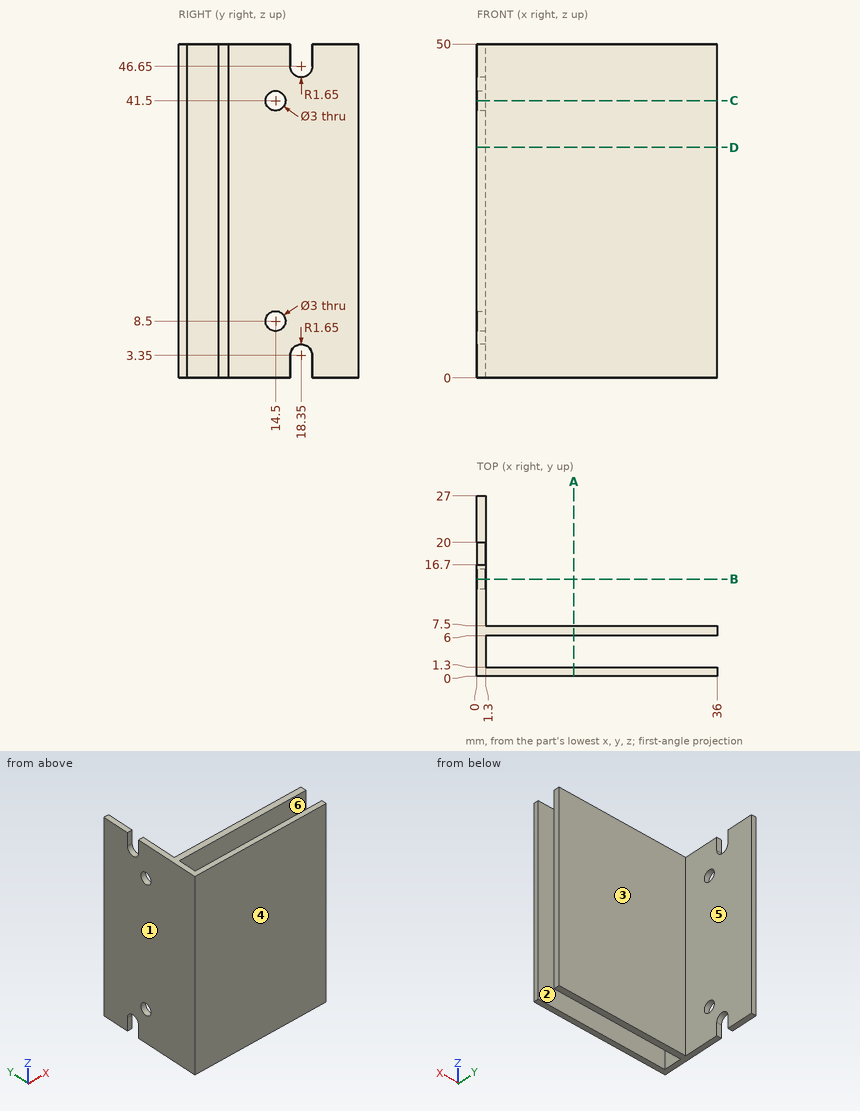
Answer from the drawing. Dimensions are ordinates in mm from the lowest x, y and z of the part. A direction names the side the tool comes from. Round coordinates to 2 decimals unless told otherwise and drop trailing zeros. Loops run counter-clockwise (first coordinate to the right, second up) from the corner with the lowest first, then second, coordinate; pieces in that order, holes last. Notation, with made-up numbers: (23.25, -2) - (61.25, -2) arc R26 cw to (61.25, 28) - close; hole circle Ø10 at (89.5, 23.25). An arc over 180 degrees is marked (long way). One line per item, written item: value.
Q1. Find section C-C on z = 41.5. Give the vertices of the cut face in (x, y), and give its area (3 significant figures).
Check values:
outline: (0, 0) - (36, 0) - (36, 1.3) - (1.3, 1.3) - (1.3, 6) - (36, 6) - (36, 7.5) - (1.3, 7.5) - (1.3, 13) - (0, 13) - close; (0, 16) - (1.3, 16) - (1.3, 27) - (0, 27) - close
area: 128 mm2
Q2. Straight lines are drawn through the part: probe 1 along Y at (x, z) = (0.65, 8.5); probe 2 along Y at (x, z) = (8.5, 45); probe 3 along X at (y, z) = (14.25, 28.5). For each, find the intervals that lie inside material, in ascending order.
Check values:
probe 1: 0 to 13, 16 to 27
probe 2: 0 to 1.3, 6 to 7.5
probe 3: 0 to 1.3
Q3. Find section A-A on x = 14.5. Give the vertices of the cut face in (y, z).
Check values:
outline: (0, 0) - (1.3, 0) - (1.3, 50) - (0, 50) - close; (6, 0) - (7.5, 0) - (7.5, 50) - (6, 50) - close
Q4. Each of these flat-tipped pins is pushed along its axis until it touches: pin 1 Ø12 at (x, z) = (18, 7.5) entering from +Y; pin 2 Ø1.5 at (y, z) = (22, 40) entering from +X. Where does it stop, or does it pass through?
Check values:
pin 1: y = 7.5
pin 2: x = 1.3
Q5. For the marked faces 5 and 6, determine the directions among +Z, -Z, +X, -X, +Y, -Y from which every point of the face is accessible in a straight line to the end or side of a thin tool.
Check values:
face 5: +Z, -Z, +X, +Y
face 6: +Z, -Z, +X
Q6. The mould has two halves that part along Y. Classify the marked faces 1, 2, 3 and 4: +Y half, -Y half, draft (parallel to the pull), parting line (faces both ways), or undercut.
Check values:
face 1: draft
face 2: undercut
face 3: +Y half
face 4: -Y half
Q7. Find section D-D on z = 34.5. Give the vertices of the cut face in (x, y).
Check values:
outline: (0, 0) - (36, 0) - (36, 1.3) - (1.3, 1.3) - (1.3, 6) - (36, 6) - (36, 7.5) - (1.3, 7.5) - (1.3, 27) - (0, 27) - close
Q8. Find section B-B on y = 14.5. Give the vertices of the cut face in (x, z).
Check values:
outline: (0, 0) - (1.3, 0) - (1.3, 7) - (0, 7) - close; (0, 10) - (1.3, 10) - (1.3, 40) - (0, 40) - close; (0, 43) - (1.3, 43) - (1.3, 50) - (0, 50) - close
